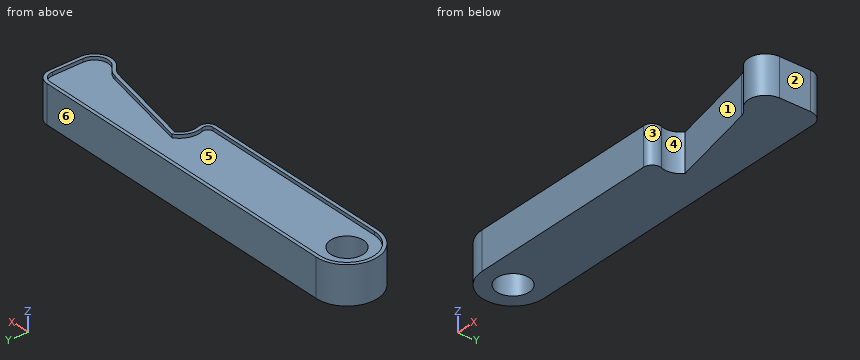
from build123d import *

# Parameters (mm, degrees)
SKETCH2_R           = 4.75
BOSS_EXTRUDE1_DEPTH = 11
CUT_EXTRUDE1_DEPTH  = 1


with BuildPart() as part:
    # Sketch2 → Boss-Extrude1 (new body)
    with BuildSketch(Plane.XY):
        with BuildLine():
            Line((0, -9), (56.97881801, -9))
            ThreePointArc((56.97881801, -9), (59.015853911, -7.949304916), (59.340646926, -5.680387791))
            ThreePointArc((59.340646926, -5.680387791), (59.261907809, -2.649407806), (60.949113688, -0.130206379))
            Line((60.949113688, -0.130206379), (87.603863211, -5.795848289))
            ThreePointArc((87.603863211, -5.795848289), (89.065679287, -6.35725315), (90.282152379, -7.343293147))
            ThreePointArc((90.282152379, -7.343293147), (95.79035777, -8.66847074), (99, -4))
            Line((99, -4), (99, 5))
            ThreePointArc((99, 5), (97.828427125, 7.828427125), (95, 9))
            Line((95, 9), (0, 9))
            ThreePointArc((0, 9), (-9, 0), (0, -9))
        make_face()
        Circle(SKETCH2_R, mode=Mode.SUBTRACT)
    extrude(amount=BOSS_EXTRUDE1_DEPTH)

    # Sketch4 → Cut-Extrude1 (cut)
    with BuildSketch(Plane.XY.offset(11)):
        with BuildLine():
            Line((60.720530375, 0.940721099), (87.811774902, -4.817700689))
            ThreePointArc((87.811774902, -4.817700689), (89.565954193, -5.491386522), (91.025721903, -6.674634517))
            ThreePointArc((91.025721903, -6.674634517), (95.432286216, -7.734776592), (98, -4))
            Line((98, -4), (98, 5))
            ThreePointArc((98, 5), (97.121320344, 7.121320344), (95, 8))
            Line((95, 8), (0, 8))
            ThreePointArc((0, 8), (-8, 0), (0, -8))
            Line((0, -8), (56.97881801, -8))
            ThreePointArc((56.97881801, -8), (58.201039551, -7.369582949), (58.39591536, -6.008232674))
            ThreePointArc((58.39591536, -6.008232674), (58.374246442, -2.137683304), (60.720530375, 0.940721099))
        make_face()
    extrude(amount=-CUT_EXTRUDE1_DEPTH, mode=Mode.SUBTRACT)


solid = part.part
CAD build for the part. Positions are in the model's coordinates, mm. Face numbers are marked on the shaded views. A direction names the side the tool comes from. Give positions to 0.01 mm unless a question says otherwise; leave off trailing zeros. Loops run counter-clockwise (first coordinate to the right, second up) from the corner with the lowest first, then second, coordinate; pieces in that order, holes last. Notation, with made-up numbers: M 31,12.5 L 85,12.5 A32 cw 85,45.5 Z; hole C 89,56.5 d7. An arc over 180 degrees is marked long. Answer in a Markdown table with one row per item. Add a question column.
Item 1: Probe probe 1 along X at (y, z) = (0, 4.5); probe 2 along Z at (x, y) = (87, 4); probe 3 along X at (y, z) = (3.75, 9.75). List the from-to ranges inside material, lowest first.
Item 2: Mould opens along Y. For the marked faces 1, 2 and 3 say: +Y half, -Y half, draft (parallel to the pull), parting line (faces both ways), or undercut.
Item 3: Band-saw the part on B-B on x = 37.5. Give the cut face in (y, z).
Item 4: Band-saw the part on D-D on x = 85. Give the cut face in (y, z), then the cut area to 3 significant figures.
Item 5: Band-saw the part on A-A on y = 2.5. Give the cut face in (x, z).
Item 6: Band-saw the part on C-C on z = 6.5. Give the cut face in (x, y), then the cut area to 3 significant figures.
Item 7: Drop flat-ended pins along their axis: P1, Ø2, axis at x = 13.5, y = 6, coming from the -Z side; P2, Ø4, axis at x = 73.5, z = 3.5, coming from the -Y side; P3, Ø0.5, axis at x = 69, z = 10.5, coming from the -Y side. Give the stop position or say it passes through.
Item 8: Tool access for the marked faces 4, 5 and 6: list every direction of +Z, -Z, +X, -X, +Y, -Y with a clear straight run to the whole face (end or side of a thin tool).
Reply:
| question | item | result |
|---|---|---|
| 1 | probe 1 | x = -9 to -4.75, 4.75 to 99 |
| 1 | probe 2 | z = 0 to 10 |
| 1 | probe 3 | x = -8.18 to -2.92, 2.92 to 99 |
| 2 | face 1 | -Y half |
| 2 | face 2 | draft |
| 2 | face 3 | undercut |
| 3 | outline | M -9,0 L 9,0 L 9,11 L 8,11 L 8,10 L -8,10 L -8,11 L -9,11 Z |
| 4 | outline | M -5.24,0 L 9,0 L 9,11 L 8,11 L 8,10 L -4.22,10 L -4.22,11 L -5.24,11 Z |
| 4 | area | 144 mm^2 |
| 5 | outline | M -8.65,0 L -4.04,0 L -4.04,10 L -7.6,10 L -7.6,11 L -8.65,11 Z; M 4.04,0 L 99,0 L 99,11 L 98,11 L 98,10 L 4.04,10 Z |
| 6 | outline | M 0,-9 L 56.98,-9 A2.5 ccw 59.34,-5.68 A5 cw 60.95,-0.13 L 87.6,-5.8 A5 cw 90.28,-7.34 A5 ccw 99,-4 L 99,5 A4 ccw 95,9 L 0,9 A9 ccw Z; hole C 0,0 d9.5 |
| 6 | area | 1,650 mm^2 |
| 7 | P1 | stops at z = 0 |
| 7 | P2 | stops at y = -3.22 |
| 7 | P3 | stops at y = -1.89 |
| 8 | face 4 | +Z, -Z |
| 8 | face 5 | +Z |
| 8 | face 6 | +Z, -Z, +X, -X, +Y |
